```python
from build123d import *

# Parameters (mm, degrees)
SKETCH4_R                    = 4
BOSS_EXTRUDE1_DEPTH          = 0.5
SKETCH5_R                    = 2
BOSS_EXTRUDE2_DEPTH          = 10.5
CHAMFER1_SIZE                = 0.5
CIRPATTERN1_COUNT            = 3
CHAMFER1_OF_CIRPATTERN1_SIZE = 0.5
BOSS_EXTRUDE3_DEPTH          = 7.5
SKETCH7_R                    = 0.75
CUT_EXTRUDE1_DEPTH           = 2
CUT_EXTRUDE2_DEPTH           = 34.686050525
CHAMFER2_SIZE                = 0.2
CHAMFER3_SIZE                = 0.5
CIRPATTERN2_COUNT            = 3
CHAMFER2_OF_CIRPATTERN2_SIZE = 0.2
CHAMFER3_OF_CIRPATTERN2_SIZE = 0.5
CHAMFER4_SIZE                = 1
FILLET1_R                    = 1


with BuildPart() as part:
    # Sketch3 → Revolve1 (revolve)
    with BuildSketch(Plane(origin=(0, 0, 0), x_dir=(0, 0, -1), z_dir=(1, 0, 0)), mode=Mode.PRIVATE) as revolve1_sk:
        Polygon((1, 13.6), (1, 12), (2.5, 12), (2.5, 10), (7, 10), (7, 21.5), (1.5, 21.5), (1.5, 20), (0, 20), (0, 13.6), align=None)
    revolve(revolve1_sk.sketch.rotate(Axis((0, 0, 0), (0, 0, -1)), 90), axis=Axis((0, 0, 0), (0, 0, -1)))

    # Sketch4 → Boss-Extrude1 (add)
    with BuildSketch(Plane(origin=(0, 0, -7), x_dir=(-1, 0, 0), z_dir=(0, 0, -1))):
        with Locations(Location((0, 16.8, 0), (0, 0, 180))):
            Circle(SKETCH4_R)
    boss_extrude1 = extrude(amount=BOSS_EXTRUDE1_DEPTH)

    # Sketch5 → Boss-Extrude2 (add)
    with BuildSketch(Plane(origin=(0, 0, -7.5), x_dir=(-1, 0, 0), z_dir=(0, 0, -1))):
        with Locations(Location((0, 16.8, 0), (0, 0, 180))):
            Circle(SKETCH5_R)
    boss_extrude2 = extrude(amount=BOSS_EXTRUDE2_DEPTH)

    # Chamfer1
    chamfer1_edges = [part.edges().sort_by_distance(p)[0] for p in [
        (-2, 16.8, -18),
    ]]
    chamfer(chamfer1_edges, length=CHAMFER1_SIZE)

    # CirPattern1: Boss-Extrude1, Boss-Extrude2 ×3 about axis
    cirpattern1_axis = Axis((0, 0, 0), (0, 0, 1))
    add([boss_extrude1.rotate(cirpattern1_axis, i * 360 / CIRPATTERN1_COUNT) for i in range(1, CIRPATTERN1_COUNT)])
    add([boss_extrude2.rotate(cirpattern1_axis, i * 360 / CIRPATTERN1_COUNT) for i in range(1, CIRPATTERN1_COUNT)])

    # Chamfer1 of CirPattern1
    chamfer1_of_cirpattern1_edges = [part.edges().sort_by_distance(p)[0] for p in [
        (-13.549226784, -10.132050808, -18),
        (15.549226784, -6.667949192, -18),
    ]]
    chamfer(chamfer1_of_cirpattern1_edges, length=CHAMFER1_OF_CIRPATTERN1_SIZE)

    # Sketch6 → Boss-Extrude3 (add)
    with BuildSketch(Plane(origin=(0, 0, -7), x_dir=(-1, 0, 0), z_dir=(0, 0, -1))):
        with BuildLine():
            ThreePointArc((-4.561681399, -8.89893605), (-6.703398823, -14.60024061), (-11.755277198, -18.001762636))
            ThreePointArc((-11.755277198, -18.001762636), (0, -21.5), (11.755277198, -18.001762636))
            ThreePointArc((11.755277198, -18.001762636), (6.703398823, -14.60024061), (4.561681399, -8.89893605))
            ThreePointArc((4.561681399, -8.89893605), (0, -10), (-4.561681399, -8.89893605))
        make_face()
    boss_extrude3 = extrude(amount=BOSS_EXTRUDE3_DEPTH)

    # Sketch7 → Cut-Extrude1 (cut)
    with BuildSketch(Plane(origin=(0, 0, -14.5), x_dir=(-1, 0, 0), z_dir=(0, 0, -1))):
        with BuildLine():
            Line((-3.105828541, -11.591109915), (-4.658742812, -17.386664873))
            ThreePointArc((-4.658742812, -17.386664873), (0, -18), (4.658742812, -17.386664873))
            Line((4.658742812, -17.386664873), (3.105828541, -11.591109915))
            ThreePointArc((3.105828541, -11.591109915), (0, -12), (-3.105828541, -11.591109915))
        make_face()
        with Locations((0, -15)):
            Circle(SKETCH7_R, mode=Mode.SUBTRACT)
    cut_extrude1 = extrude(amount=-CUT_EXTRUDE1_DEPTH, mode=Mode.SUBTRACT)

    # Sketch7<3> → Cut-Extrude2 (cut, through all)
    with BuildSketch(Plane(origin=(0, 0, -14.5), x_dir=(-1, 0, 0), z_dir=(0, 0, -1))):
        with BuildLine():
            ThreePointArc((0.75, -15), (0.530330086, -14.469669914), (0, -14.25))
            Line((0, -14.25), (0, -15.75))
            ThreePointArc((0, -15.75), (0.530330086, -15.530330086), (0.75, -15))
        make_face()
        with BuildLine():
            Line((0, -15.75), (0, -14.25))
            ThreePointArc((0, -14.25), (-0.75, -15), (0, -15.75))
        make_face()
    cut_extrude2 = extrude(amount=-CUT_EXTRUDE2_DEPTH, mode=Mode.SUBTRACT)

    # Chamfer2
    chamfer2_edges = [part.edges().sort_by_distance(p)[0] for p in [
        (0, -15.75, -12.5),
    ]]
    chamfer(chamfer2_edges, length=CHAMFER2_SIZE)

    # Chamfer3
    chamfer3_edges = [part.edges().sort_by_distance(p)[0] for p in [
        (0, -12, -14.5),
        (3.882285677, -14.488887394, -14.5),
        (0, -18, -14.5),
        (-3.882285677, -14.488887394, -14.5),
    ]]
    chamfer(chamfer3_edges, length=CHAMFER3_SIZE)

    # CirPattern2: Boss-Extrude3, Cut-Extrude1, Cut-Extrude2 ×3 about axis
    cirpattern2_axis = Axis((0, 0, 0), (0, 0, 1))
    add([boss_extrude3.rotate(cirpattern2_axis, i * 360 / CIRPATTERN2_COUNT) for i in range(1, CIRPATTERN2_COUNT)])
    add([cut_extrude1.rotate(cirpattern2_axis, i * 360 / CIRPATTERN2_COUNT) for i in range(1, CIRPATTERN2_COUNT)], mode=Mode.SUBTRACT)
    add([cut_extrude2.rotate(cirpattern2_axis, i * 360 / CIRPATTERN2_COUNT) for i in range(1, CIRPATTERN2_COUNT)], mode=Mode.SUBTRACT)

    # Chamfer2 of CirPattern2
    chamfer2_of_cirpattern2_edges = [part.edges().sort_by_distance(p)[0] for p in [
        (13.63990011, 7.875, -12.5),
        (-13.63990011, 7.875, -12.5),
    ]]
    chamfer(chamfer2_of_cirpattern2_edges, length=CHAMFER2_OF_CIRPATTERN2_SIZE)

    # Chamfer3 of CirPattern2
    chamfer3_of_cirpattern2_edges = [part.edges().sort_by_distance(p)[0] for p in [
        (10.392304845, 6, -14.5),
        (10.606601718, 10.606601718, -14.5),
        (15.588457268, 9, -14.5),
        (14.488887394, 3.882285677, -14.5),
        (-10.392304845, 6, -14.5),
        (-14.488887394, 3.882285677, -14.5),
        (-15.588457268, 9, -14.5),
        (-10.606601718, 10.606601718, -14.5),
    ]]
    chamfer(chamfer3_of_cirpattern2_edges, length=CHAMFER3_OF_CIRPATTERN2_SIZE)

    # Chamfer4
    chamfer4_edges = [part.edges().sort_by_distance(p)[0] for p in [
        (-20, 0, 0),
    ]]
    chamfer(chamfer4_edges, length=CHAMFER4_SIZE)

    # Fillet1
    # the kernel refuses this fillet: 1 mm, written as the material it takes off along each edge
    with BuildSketch(Plane(origin=(21.467622355, -1.179487364, -7), x_dir=(0.006387197521753035, 0.9999796016458627, 0), z_dir=(0, 0, -1)), Plane(origin=(-9.712345156, 19.18125, -7), x_dir=(-0.8692013370524373, -0.49445832551010344, 0), z_dir=(0, 0, -1)), Plane(origin=(-11.755277198, -18.001762636, -7), x_dir=(0.862814139530684, -0.5055212761357581, 0), z_dir=(0, 0, -1))) as fillet1_piece_1:
        with BuildLine():
            CenterArc((2.036209541, -0.998824096), FILLET1_R, 87.221143718, 125.050734124)
            ThreePointArc((1.190685537, -1.532761506), (0.632617432, -0.737424909), (0, 0))
            ThreePointArc((0, 0), (1.04234536, 0.025281931), (2.084690721, 0))
        make_face()
    extrude(amount=12.711726802, mode=Mode.SUBTRACT)
    with BuildSketch(Plane(origin=(9.987545385, 0.49893605, -7), x_dir=(0.9173175626436978, 0.3981563628342837, 0), z_dir=(0, 0, -1)), Plane(origin=(-5.425863987, 8.4, -7), x_dir=(-0.8034723062147525, 0.5953421311699238, 0), z_dir=(0, 0, -1)), Plane(origin=(-4.561681399, -8.89893605, -7), x_dir=(-0.113845256428944, -0.9934984940042073, 0), z_dir=(0, 0, -1))) as fillet1_piece_2:
        with BuildLine():
            CenterArc((1.346819148, -0.99794128), FILLET1_R, 93.677145319, 99.571657965)
            ThreePointArc((0.373435102, -1.22712134), (0.20641295, -0.607567006), (0, 0))
            ThreePointArc((0, 0), (0.641342451, -0.020587199), (1.282684903, 0))
        make_face()
    extrude(amount=10.706712257, mode=Mode.SUBTRACT)
    with BuildSketch(Plane(origin=(5.425863987, 8.4, -7), x_dir=(0.8034723062147457, 0.595342131169933, 0), z_dir=(0, 0, -1)), Plane(origin=(-9.987545385, 0.49893605, -7), x_dir=(-0.9173175626437021, 0.3981563628342733, 0), z_dir=(0, 0, -1)), Plane(origin=(4.561681399, -8.89893605, -7), x_dir=(0.11384525642895783, -0.9934984940042058, 0), z_dir=(0, 0, -1))) as fillet1_piece_3:
        with BuildLine():
            CenterArc((1.346819148, 0.99794128), FILLET1_R, 166.751196715, 99.571657965)
            ThreePointArc((0.373435102, 1.22712134), (0.20641295, 0.607567006), (0, 0))
            ThreePointArc((0, 0), (0.641342451, 0.020587199), (1.282684903, 0))
        make_face()
    extrude(amount=10.706712257, mode=Mode.SUBTRACT)
    with BuildSketch(Plane(origin=(9.712345156, 19.18125, -7), x_dir=(0.8692013370524435, -0.4944583255100922, 0), z_dir=(0, 0, -1)), Plane(origin=(-21.467622355, -1.179487364, -7), x_dir=(-0.006387197521766656, 0.9999796016458625, 0), z_dir=(0, 0, -1)), Plane(origin=(11.755277198, -18.001762636, -7), x_dir=(-0.8628141395306765, -0.5055212761357707, 0), z_dir=(0, 0, -1))) as fillet1_piece_4:
        with BuildLine():
            CenterArc((2.036209541, 0.998824096), FILLET1_R, 147.728122158, 125.050734124)
            ThreePointArc((1.190685537, 1.532761506), (0.632617432, 0.737424909), (0, 0))
            ThreePointArc((0, 0), (1.04234536, -0.025281931), (2.084690721, 0))
        make_face()
    extrude(amount=12.711726802, mode=Mode.SUBTRACT)


solid = part.part
```
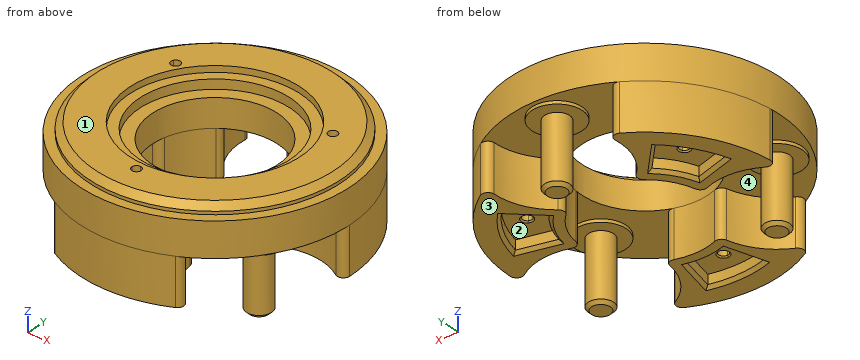
Can you work these out from the model? Positions are in its coordinate system, mm. Face numbers are marked on the shaded views. A direction names the side the tool comes from. Round coordinates to 2 decimals unless told otherwise and drop trailing zeros. Order: outer loops, then holes, each group sorted by start corner. A loop starts at its lowest first (then second) coordinate and runs counter-clockwise, first axis right, second up.
(1) We'd pull the mould along Y, two halves only. Please class the marked faces 3 and 4: +Y half, -Y half, draft (parallel to the pull), parting line (faces both ways), or undercut.
Results are:
face 3: draft
face 4: undercut
(2) I'm going to push flat-ended pins straight in: pin 1 (6 mm diameter, centred on y = -2, z = -9.5, fed in from +X); pin 2 (7 mm diameter, centred on x = 5, y = -1.5, fed in from +Z); pin 3 (8 mm diameter, centred on y = -5, z = -13.5, fed in from +X); pin 4 (21.5 mm diameter, centred on x = 0, y = 0, fed in from -Z). Where does each tip first touch, or does it pass through?
Results are:
pin 1: stops at x = 21.5
pin 2: passes through
pin 3: stops at x = 16.55
pin 4: stops at z = -14.5
(3) On a 3-axis mill with a long thin cutter (end or side, diameter ignored), from which of +Z, -Z, +X, -X, +Y, -Y can I reach the whole of each face in a straight line? I mean the marked faces 1 and 2. Say none if no direction works.
Results are:
face 1: +Z, +X, -X, +Y, -Y
face 2: -Z
(4) If we section it at C-C (z = -16): Please give me the cut outline in (x, y).
Results are:
outline: circle Ø4 at (-14.55, -8.4); circle Ø4 at (0, 16.8); circle Ø4 at (14.55, -8.4)
(5) If we section it at B-B (z = -11.25): Count the separate pieces of the cut face and the enclosed holes in it, plus the area to 3 significant figures.
Results are:
separate pieces: 6
enclosed holes: 3
area: 530 mm2
(6) If we section it at A-A (z = -3.25): Please give me the cut outline in (x, y) (3 decimals).
Results are:
outline: circle Ø43 at (0, 0); hole circle Ø1.5 at (-12.99, 7.5); hole circle Ø20 at (0, 0); hole circle Ø1.5 at (0, -15); hole circle Ø1.5 at (12.99, 7.5)
(7) If I drill on L1, parallel to Y at x = 0, z = -4.5; L2, parallel to Y at x = 0, z = -2.2; L3, parallel to X at y = 8, z = -8.75, over which ranges is the centre line in solid material (lowest first)?
Results are:
L1: y = -21.5 to -15.75, -14.25 to -10, 10 to 21.5
L2: y = -21.5 to -15.75, -14.25 to -12, 12 to 21.5
L3: x = -19.96 to -13.55, -12.43 to -6.19, 6.19 to 12.43, 13.55 to 19.96
